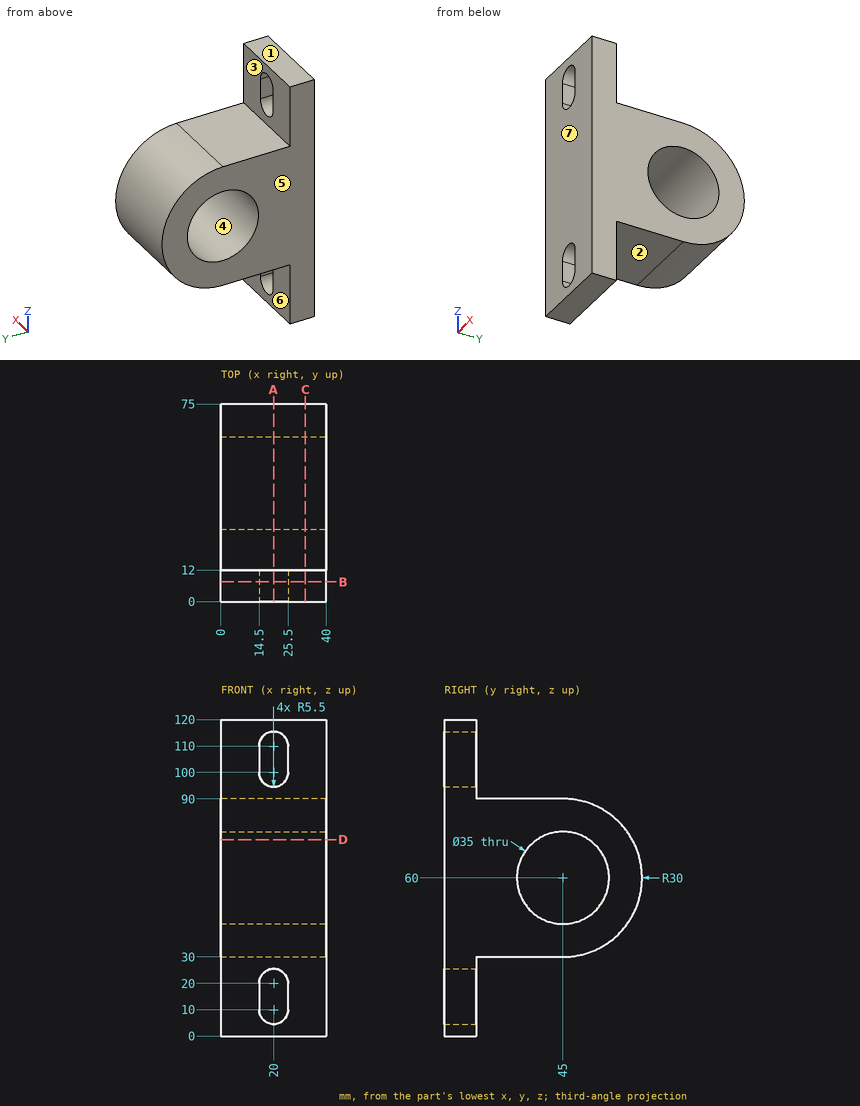
Check sheet for the drawn part. Datum: minimum x, y, z corner. Units: mm. A direction names the side the tool comes from. Give positions to 0.01 mm unless a question says otherwise; leave off trailing zeros. Order: outer loops, then holes, each group sorted by start corner. A loop starts at its lowest first (then second) coordinate and runs counter-clockwise, first axis right, second up. Notation, with made-up numbers: (51.25, 26) -> (74.25, 26) arc R27 cw to (74.25, 61) -> close; hole circle Ø10 at (-2.5, -4). An arc over 180 degrees is marked (long way). One line per item, written item: value.
(1) Gauge pin test, flat ends, axial feed: pin 1 (1 mm diameter, centred on x = 9, y = 21, fed in from +Z); pin 2 (24 mm diameter, centred on x = 15.5, z = 22.5, fed in from +Y); pin 3 (1.5 mm diameter, centred on x = 28.5, y = 59.5, fed in from -Z). Record the tip position at first contact, or that the pin passes through.
Final values:
pin 1: z = 90
pin 2: y = 60.8
pin 3: z = 33.34
(2) Draft check along Y on the marked faces 4, 5, 6 and 7. Enter one of: pulls with the +Y half, pulls with the -Y half, needs draft (parallel to the pull), parting line crosses it, or undercut.
Final values:
face 4: undercut
face 5: needs draft
face 6: pulls with the +Y half
face 7: pulls with the -Y half
(3) Sectioned sample at A-A on x = 20. Record the cut outline in (y, z), then the cut area to 3 significant figures.
Final values:
outline: (0, 0) -> (12, 0) -> (12, 4.5) -> (0, 4.5) -> close; (0, 25.5) -> (12, 25.5) -> (12, 30) -> (45, 30) arc R30 ccw to (45, 90) -> (12, 90) -> (12, 94.5) -> (0, 94.5) -> close; (0, 115.5) -> (12, 115.5) -> (12, 120) -> (0, 120) -> close; hole circle Ø35 at (45, 60)
area: 3,370 mm^2
(4) Sectioned sample at D-D on z = 74.5. Record the cut outline in (x, y), then the cut area to 3 significant figures.
Final values:
outline: (0, 0) -> (40, 0) -> (40, 35.2) -> (0, 35.2) -> close; (0, 54.8) -> (40, 54.8) -> (40, 71.26) -> (0, 71.26) -> close
area: 2,070 mm^2
(5) Sectioned sample at B-B on y = 7.5. Record the cut outline in (x, z), then the cut area to 3 significant figures.
Final values:
outline: (0, 0) -> (40, 0) -> (40, 120) -> (0, 120) -> close; hole (14.5, 10) arc R5.5 ccw to (25.5, 10) -> (25.5, 20) arc R5.5 ccw to (14.5, 20) -> close; hole (14.5, 100) arc R5.5 ccw to (25.5, 100) -> (25.5, 110) arc R5.5 ccw to (14.5, 110) -> close
area: 4,390 mm^2
(6) Scan lines: line 1 along Y through (x, z) = (22, 60); line 2 along Z through (x, y) = (4, 47); line 3 along Y through (x, z) = (35.5, 107.5). Record each from-to range of solid material in increasing order. Write a range as [from, to].
Final values:
line 1: [0, 27.5], [62.5, 75]
line 2: [30.07, 42.61], [77.39, 89.93]
line 3: [0, 12]
(7) Tool access check on the marked faces 1, 2 and 3. Record the directions out of +Z, -Z, +X, -X, +Y, -Y that give a thin tool (end or side, any length) a straight path to the whole face; none if there is none.
Final values:
face 1: +Z, +X, -X, +Y, -Y
face 2: -Z, +X, -X, +Y
face 3: +Z, +X, -X, +Y
(8) Sectioned sample at C-C on x = 32. Record the cut outline in (y, z), then the cut area to 3 significant figures.
Final values:
outline: (0, 0) -> (12, 0) -> (12, 30) -> (45, 30) arc R30 ccw to (45, 90) -> (12, 90) -> (12, 120) -> (0, 120) -> close; hole circle Ø35 at (45, 60)
area: 3,870 mm^2
